Could you check a few things on this model? Use its own coordinates, in mm. A direction names the side the tool comes from. Coordinates: 2 decimals unless noted, no trailing zeros. Order: outer loops, then holes, each group sorted by start corner. A loop starts at its lowest first (then second) coordinate and runs counter-clockwise, first axis right, second up. Notation, with made-up numbers: (-9, 75.5) -> (-4, 75.5) arc R25 ccw to (-4, 91.5) -> close; hole circle Ø8 at (-40, 26.25). An arc over 180 degrees is marked (long way). Use a Markdown table: item, result. Add a question column.
1) Which directions (+Z, -Z, +X, -X, +Y, -Y) give clear straight access to the entire face, cutting with the end or side of a thin tool? Please do faces 1 (the cylindrical face through (0.86, 70.86, -4.39)), 2 (the flat face through (0, 1, -3.8)).
2) Thinking about a two-plate mould opening in Y: for faces 3 (the flat face through (0, 1, 3.8)), 4 (the flat face through (0, -74.51, 4)), 5 (the cylindrical face through (0.86, -70.86, 4.41)), which applies, +Y half, -Y half, draft (parallel to the pull), parting line (faces both ways), or undercut?
3) If we section it at D-D (y = 30.5): Write out the boundary of the cut face in (x, z).
4) If we section it at C-C (x = -3.5): Write out the boundary of the cut face in (y, z), plus the area to 3 significant figures.
5) If we section it at B-B (z = -2): Write out the boundary of the cut face in (x, y).
6) If we section it at A-A (y = -37.5): Write out the boundary of the cut face in (x, z).
7) If I drill on L1, parallel to Z at x = 3.75, y = -40.5; L2, parallel to X at y = 17.5, z = -1.5; L3, parallel to X at y = -37.5, z = 4.5, over which ranges is the centre line in solid material (lowest first)? Write a range as [from, to].
```python
from build123d import *

# Parameters (mm, degrees)
SKETCH_1_W          = 15
SKETCH_1_H          = 10
SKETCH_1_W_2        = 12.6
SKETCH_1_H_2        = 7.6
EXTRUDE_1_DEPTH     = 74.51
SKETCH_3_R          = 1.6
CUT_EXTRUDE_1_DEPTH = 10
SKETCH_4_R          = 1.6
CUT_EXTRUDE_2_DEPTH = 10


with BuildPart() as part:
    # ｽｹｯﾁ1 → ﾎﾞｽ - 押し出し1 (new, symmetric)
    with BuildSketch(Plane(origin=(0, 0, 0), x_dir=(1, 0, 0), z_dir=(0, 1, 0))):
        Rectangle(SKETCH_1_W, SKETCH_1_H)
        Rectangle(SKETCH_1_W_2, SKETCH_1_H_2, mode=Mode.SUBTRACT)
    extrude(amount=EXTRUDE_1_DEPTH, both=True)

    # ｽｹｯﾁ3 → ｶｯﾄ - 押し出し1 (cut)
    with BuildSketch(Plane.XY.offset(5)):
        with Locations((0, 49.51)):
            Circle(SKETCH_3_R)
        with Locations((0, 69.51)):
            Circle(SKETCH_3_R)
    cut_extrude_1 = extrude(amount=-CUT_EXTRUDE_1_DEPTH, mode=Mode.SUBTRACT)

    # ﾐﾗｰ1: ｶｯﾄ - 押し出し1 across plane
    add(cut_extrude_1.mirror(Plane.ZX), mode=Mode.SUBTRACT)

    # ｽｹｯﾁ4 → ｶｯﾄ - 押し出し2 (cut)
    with BuildSketch(Plane(origin=(0, 0, -5), x_dir=(-1, 0, 0), z_dir=(0, 0, -1))):
        with Locations((0, 37.5)):
            Circle(SKETCH_4_R)
        with Locations(Location((0, -37.5, 0), (0, 0, 180))):
            Circle(SKETCH_4_R)
    extrude(amount=-CUT_EXTRUDE_2_DEPTH, mode=Mode.SUBTRACT)


solid = part.part
```
Answer sheet:
| question | item | result |
|---|---|---|
| 1 | face 1 | +Z, -Z |
| 1 | face 2 | +Y, -Y |
| 2 | face 3 | draft |
| 2 | face 4 | -Y half |
| 2 | face 5 | undercut |
| 3 | outline | (-7.5, -5) -> (7.5, -5) -> (7.5, 5) -> (-7.5, 5) -> close; hole (-6.3, -3.8) -> (6.3, -3.8) -> (6.3, 3.8) -> (-6.3, 3.8) -> close |
| 4 | outline | (-74.51, -5) -> (74.51, -5) -> (74.51, -3.8) -> (-74.51, -3.8) -> close; (-74.51, 3.8) -> (74.51, 3.8) -> (74.51, 5) -> (-74.51, 5) -> close |
| 4 | area | 358 mm2 |
| 5 | outline | (-7.5, -74.51) -> (-6.3, -74.51) -> (-6.3, 74.51) -> (-7.5, 74.51) -> close; (6.3, -74.51) -> (7.5, -74.51) -> (7.5, 74.51) -> (6.3, 74.51) -> close |
| 6 | outline | (-7.5, -5) -> (-1.6, -5) -> (-1.6, -3.8) -> (-6.3, -3.8) -> (-6.3, 3.8) -> (-1.6, 3.8) -> (-1.6, 5) -> (-7.5, 5) -> close; (1.6, -5) -> (7.5, -5) -> (7.5, 5) -> (1.6, 5) -> (1.6, 3.8) -> (6.3, 3.8) -> (6.3, -3.8) -> (1.6, -3.8) -> close |
| 7 | L1 | [-5, -3.8], [3.8, 5] |
| 7 | L2 | [-7.5, -6.3], [6.3, 7.5] |
| 7 | L3 | [-7.5, -1.6], [1.6, 7.5] |
